```python
from build123d import *

# Parameters (mm, degrees)
BOSS_EXTRUDE1_DEPTH = 4.75


with BuildPart() as part:
    # Sketch1 → Boss-Extrude1 (new body)
    with BuildSketch(Plane.XY):
        with BuildLine():
            Line((28.105438967, -10.25), (28.105438967, -15.25))
            Line((28.105438967, -15.25), (-71.894561033, -15.25))
            Line((-71.894561033, -15.25), (-71.894561033, -10.25))
            ThreePointArc((-71.894561033, -10.25), (-71.601667814, -9.542893219), (-70.894561033, -9.25))
            Line((-70.894561033, -9.25), (-53.894561033, -9.25))
            Line((-53.894561033, -9.25), (-53.894561033, -5.85))
            Line((-53.894561033, -5.85), (-70.894561033, -5.85))
            ThreePointArc((-70.894561033, -5.85), (-71.601667814, -5.557106781), (-71.894561033, -4.85))
            Line((-71.894561033, -4.85), (-71.894561033, 5.15))
            ThreePointArc((-71.894561033, 5.15), (-71.601667814, 5.857106781), (-70.894561033, 6.15))
            Line((-70.894561033, 6.15), (-54.894561033, 6.15))
            Line((-54.894561033, 6.15), (-54.894561033, 9.55))
            Line((-54.894561033, 9.55), (-70.894561033, 9.55))
            ThreePointArc((-70.894561033, 9.55), (-71.601667814, 9.842893219), (-71.894561033, 10.55))
            Line((-71.894561033, 10.55), (-71.894561033, 15.55))
            Line((-71.894561033, 15.55), (28.105438967, 15.55))
            Line((28.105438967, 15.55), (28.105438967, 10.55))
            ThreePointArc((28.105438967, 10.55), (27.812545748, 9.842893219), (27.105438967, 9.55))
            Line((27.105438967, 9.55), (11.105438967, 9.55))
            Line((11.105438967, 9.55), (11.105438967, 6.15))
            Line((11.105438967, 6.15), (27.105438967, 6.15))
            ThreePointArc((27.105438967, 6.15), (27.812545748, 5.857106781), (28.105438967, 5.15))
            Line((28.105438967, 5.15), (28.105438967, -4.85))
            ThreePointArc((28.105438967, -4.85), (27.812545748, -5.557106781), (27.105438967, -5.85))
            Line((27.105438967, -5.85), (10.105438967, -5.85))
            Line((10.105438967, -5.85), (10.105438967, -9.25))
            Line((10.105438967, -9.25), (27.105438967, -9.25))
            ThreePointArc((27.105438967, -9.25), (27.812545748, -9.542893219), (28.105438967, -10.25))
        make_face()
    extrude(amount=BOSS_EXTRUDE1_DEPTH)


solid = part.part
```
Check sheet for the modelled part. Datum: model origin and axes. Units: mm. A direction names the side the tool comes from. Give positions to 0.01 mm unless a question says otherwise; leave off trailing zeros. Order: outer loops, then holes, each group sorted by start corner. A loop starts at its lowest first (then second) coordinate and runs counter-clockwise, first axis right, second up. Notation, with made-up numbers: M -35.75,83 L 5.25,83 A34 cw 5.25,122 Z; hole C 87.25,87.5 d6. An arc over 180 degrees is marked long. Answer in a Markdown table with one row per item. Add a question column.
Q1. Release check for a two-part mould opening along Y. For faces 1 (the flat face through (28.105, 0, 2)), 2 (the flat face through (-23, 15.55, 2)), 3 (the flat face through (19, 9.55, 2)) record: released by +Y, released by -Y, zero draft, split by the parting line, or undercut.
Q2. Gauge pin test, flat ends, axial feed: pin 1 Ø1.7 at (y, z) = (7.5, 3.5) entering from -X; pin 2 Ø1 at (y, z) = (7.5, 2) entering from +X; pin 3 Ø1 at (y, z) = (-9, 2.5) entering from +X. Record the tip position at first contact, or that the pin passes through.
Q3. Sectioned sample at C-C, the plane y = 7. Record the boundary of the cut face in (x, z), and give its area (4 significant figures).
Q4. Sectioned sample at B-B, the plane z = 3.35. Record the boundary of the cut face in (x, y), and give its area (3 significant figures).
Q5. Sectioned sample at A-A, the plane x = 13. Record the boundary of the cut face in (y, z), and give its area (3 significant figures).
Q6. Access from +Z, -Z, +X, -X, +Y, -Y to the whole of each face (thin tool, end or side, straight path). Record for faces 4 (the flat face through (-71.895, 13, 2)), 5 (the flat face through (18, -9.25, 2)), 6 (the flat face through (-63, -9.25, 2)).
Q7. Thickness scan on L1, parallel to Y at x = -57, z = 3.3; L2, parallel to X at y = 7, z = 3.6. Record the ranges inside material, lowest first.
Verdict:
| question | item | result |
|---|---|---|
| 1 | face 1 | zero draft |
| 1 | face 2 | released by +Y |
| 1 | face 3 | undercut |
| 2 | pin 1 | x = -54.89 |
| 2 | pin 2 | x = 11.11 |
| 2 | pin 3 | x = 27.77 |
| 3 | outline | M -54.89,0 L 11.11,0 L 11.11,4.75 L -54.89,4.75 Z |
| 3 | area | 313.5 mm² |
| 4 | outline | M -71.89,-15.25 L 28.11,-15.25 L 28.11,-10.25 A1 ccw 27.11,-9.25 L 10.11,-9.25 L 10.11,-5.85 L 27.11,-5.85 A1 ccw 28.11,-4.85 L 28.11,5.15 A1 ccw 27.11,6.15 L 11.11,6.15 L 11.11,9.55 L 27.11,9.55 A1 ccw 28.11,10.55 L 28.11,15.55 L -71.89,15.55 L -71.89,10.55 A1 ccw -70.89,9.55 L -54.89,9.55 L -54.89,6.15 L -70.89,6.15 A1 ccw -71.89,5.15 L -71.89,-4.85 A1 ccw -70.89,-5.85 L -53.89,-5.85 L -53.89,-9.25 L -70.89,-9.25 A1 ccw -71.89,-10.25 Z |
| 4 | area | 2,840 mm² |
| 5 | outline | M -15.25,0 L -9.25,0 L -9.25,4.75 L -15.25,4.75 Z; M -5.85,0 L 6.15,0 L 6.15,4.75 L -5.85,4.75 Z; M 9.55,0 L 15.55,0 L 15.55,4.75 L 9.55,4.75 Z |
| 5 | area | 114 mm² |
| 6 | face 4 | +Z, -Z, -X, +Y, -Y |
| 6 | face 5 | +Z, -Z, +X |
| 6 | face 6 | +Z, -Z, -X |
| 7 | L1 | -15.25 to -9.25, -5.85 to 6.15, 9.55 to 15.55 |
| 7 | L2 | -54.89 to 11.11 |
